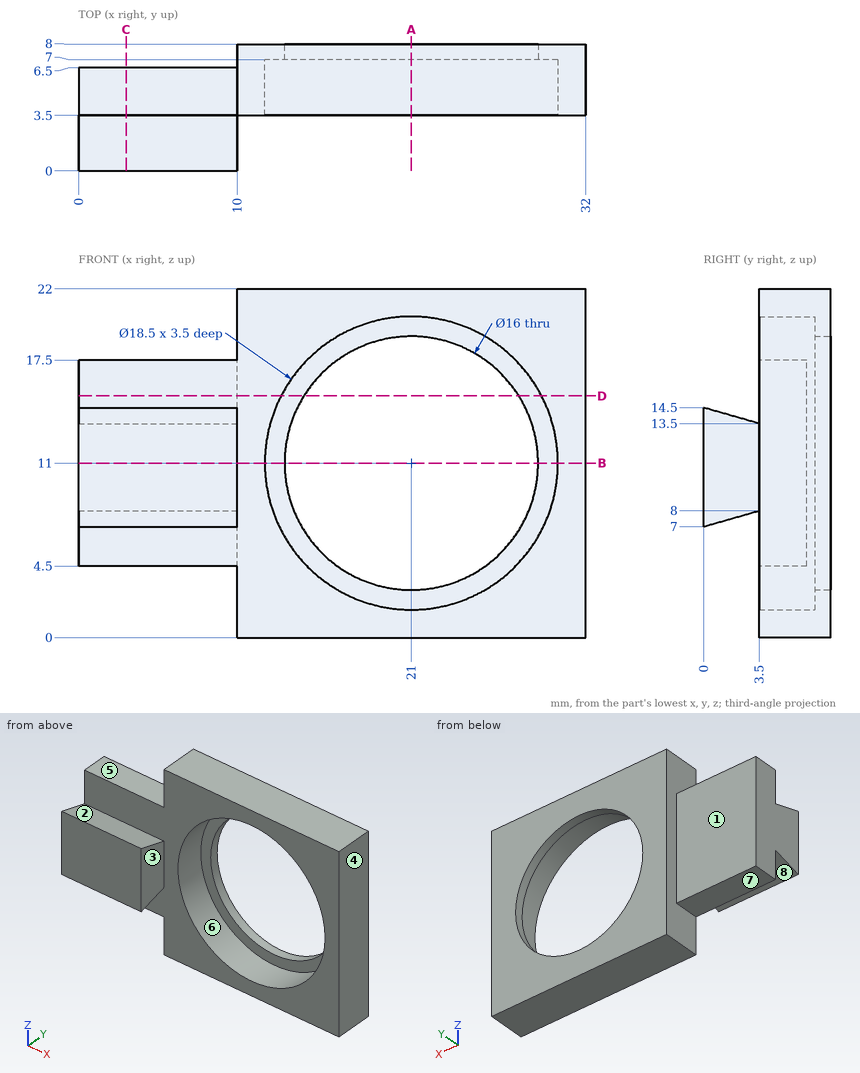
Verification items for this drawing (mm, ordinates from the low corner). A direction names the side the tool comes from. Coordinates: 2 decimals unless noted, no trailing zeros. Write each loop counter-clockwise with the first axis right and the second up, starting at its lowest first coordinate (ties: lowest second). Pieces come first, ordered by that corner, then holes. Notation, with made-up numbers: M 62.25,59 L 106.25,59 A7 ccw 106.25,67 Z; hole C -33.5,70.5 d9. An arc over 180 degrees is marked long. Answer as a JSON object with one key per item and string values.
1. Section check B-B, the plane z = 11. Enter the section's corners in (x, y), plus the area to 4 significant figures.
Answers below:
{"outline": "M 0,0 L 10,0 L 10,3.5 L 11.75,3.5 L 11.75,7 L 13,7 L 13,8 L 10,8 L 10,6.5 L 0,6.5 Z; M 29,7 L 30.25,7 L 30.25,3.5 L 32,3.5 L 32,8 L 29,8 Z", "area": "83.25 mm²"}
2. Tool access check on the marked faces 4, 5, 6, 7 and 8. Record the directions out of +Z, -Z, +X, -X, +Y, -Y that give a thin tool (end or side, any length) a straight path to the whole face; none if there is none.
Answers below:
{"face 4": "+Z, -Z, +X, +Y, -Y", "face 5": "+Z, -X, +Y, -Y", "face 6": "-Y", "face 7": "-Z, -X, +Y, -Y", "face 8": "-Z, +X, -X"}
3. Scan lines: L1, parallel to Z at x = 21, y = 5.1; L2, parallel to Z at x = 21, y = 7.8; L3, parallel to X at y = 2.5, z = 10.5. Record each from-to range of solid material in increasing order.
Answers below:
{"L1": "z = 0 to 1.75, 20.25 to 22", "L2": "z = 0 to 3, 19 to 22", "L3": "x = 0 to 10"}
4. Section check A-A, the plane x = 21. Enter the section's corners in (y, z).
Answers below:
{"outline": "M 3.5,0 L 8,0 L 8,3 L 7,3 L 7,1.75 L 3.5,1.75 Z; M 3.5,20.25 L 7,20.25 L 7,19 L 8,19 L 8,22 L 3.5,22 Z"}
5. Section check D-D, the plane z = 15.25. Enter the section's corners in (x, y), plus the area to 3 significant figures.
Answers below:
{"outline": "M 0,3.5 L 12.78,3.5 L 12.78,7 L 14.22,7 L 14.22,8 L 10,8 L 10,6.5 L 0,6.5 Z; M 27.78,7 L 29.22,7 L 29.22,3.5 L 32,3.5 L 32,8 L 27.78,8 Z", "area": "57.9 mm²"}
6. Go/stop test with flat-tipped pins: pin 1 Ø1.5 at (x, y) = (5.5, 5.5) entering from +Z; pin 2 Ø3 at (y, z) = (1, 12.5) entering from +X; pin 3 Ø0.9 at (x, y) = (5, 5) entering from -Z. Record where each tip stops, or that it passes through.
Answers below:
{"pin 1": "stops at z = 17.5", "pin 2": "stops at x = 10", "pin 3": "stops at z = 4.5"}
7. Section check C-C, the plane x = 3. Enter the section's corners in (y, z), plus the area to 4 significant figures.
Answers below:
{"outline": "M 0,7 L 3.5,8 L 3.5,4.5 L 6.5,4.5 L 6.5,17.5 L 3.5,17.5 L 3.5,13.5 L 0,14.5 Z", "area": "61.75 mm²"}
8. Draft check along Y on the marked faces 1, 2 and 3. Enter one of: released by +Y, released by -Y, zero draft, split by the parting line, or undercut.
Answers below:
{"face 1": "released by +Y", "face 2": "undercut", "face 3": "zero draft"}
